from build123d import *

# Parameters (mm, degrees)
F0_R     = 171.45
F0_R_2   = 19.05
F0_R_3   = 6.35
F1_DEPTH = 31.75
F2_DEPTH = 6.35


with BuildPart() as f1:
    # F0 (on Front) → F1 (new body)
    with BuildSketch(Plane.XZ):
        Circle(F0_R)
        with Locations((0, -50.8)):
            Circle(F0_R_2, mode=Mode.SUBTRACT)
        with Locations((-50.8, 0)):
            Circle(F0_R_2, mode=Mode.SUBTRACT)
        Circle(F0_R_3, mode=Mode.SUBTRACT)
        with Locations((50.8, 0)):
            Circle(F0_R_2, mode=Mode.SUBTRACT)
        with Locations((0, 50.8)):
            Circle(F0_R_2, mode=Mode.SUBTRACT)
    extrude(amount=F1_DEPTH)

    # F0 (on Front) → F2 (join)
    with BuildSketch(Plane.XZ):
        with Locations((0, 50.8)):
            Circle(F0_R_2)
        with Locations((50.8, 0)):
            Circle(F0_R_2)
        with Locations((-50.8, 0)):
            Circle(F0_R_2)
        with Locations((0, -50.8)):
            Circle(F0_R_2)
    extrude(amount=F2_DEPTH)


solid = f1.part
Read the model definition and answer for the solid it produces. Units are mm, in the model's axes. A direction names the side the tool comes from. Coordinates: 2 decimals unless noted, no trailing zeros. Loops run counter-clockwise (first coordinate to the right, second up) from the corner with the lowest first, then second, coordinate; pieces in that order, holes last. Notation, with made-up numbers: (-2, 86) -> (5, 86) arc R21 cw to (5, 107) -> close; hole circle Ø4 at (46.5, 80.5). An arc over 180 degrees is marked (long way). Answer in a Markdown table with one row per item.
Item 1: For a pull along X with two mould halves and no side action, classify faces 3 (the cylindrical face through (92.17, -15.653, 144.567)), 4 (the cylindrical face through (-4.13, -18.872, 32.203)), 5 (the flat face through (36, 0, 2)) as released by +X, released by -X, zero draft, split by the parting line, or undercut.
Returned:
| item | result |
|---|---|
| face 3 | split by the parting line |
| face 4 | undercut |
| face 5 | zero draft |
Item 2: For faces 1 (the flat face through (36, -31.75, -36)), 2 (the flat face through (0, -6.35, -51)), determine the directions among +Z, -Z, +X, -X, +Y, -Y from which every point of the face is accessible in a straight line to the end or side of a thin tool.
Returned:
| item | result |
|---|---|
| face 1 | +Z, -Z, +X, -X, -Y |
| face 2 | -Y |
Item 3: A cutting plane is placed at C-C on z = 50.8. Determine the outline of the cut face in (x, y).
Returned:
| item | result |
|---|---|
| outline | (-163.75, -31.75) -> (-19.05, -31.75) -> (-19.05, -6.35) -> (19.05, -6.35) -> (19.05, -31.75) -> (163.75, -31.75) -> (163.75, 0) -> (-163.75, 0) -> close |
Item 4: Each of these flat-tipped pins is pushed along its axis until it touches: P1, Ø19, axis at x = -8, z = -53, coming from the -Y side; P2, Ø10, axis at y = -13.5, z = 23, coming from the -X side; P3, Ø2, axis at x = 87, y = -12, coming from the +Z side. Where does it stop, or does it pass through?
Returned:
| item | result |
|---|---|
| P1 | stops at y = -6.35 |
| P2 | stops at x = -170.5 |
| P3 | stops at z = 148.32 |
Item 5: A cutting plane is placed at B-B on y = -17. Determine the outline of the cut face in (x, z).
Returned:
| item | result |
|---|---|
| outline | circle Ø342.9 at (0, 0); hole circle Ø38.1 at (-50.8, 0); hole circle Ø38.1 at (0, -50.8); hole circle Ø38.1 at (0, 50.8); hole circle Ø12.7 at (0, 0); hole circle Ø38.1 at (50.8, 0) |
Item 6: Straight lines are drawn through the part: line 1 along Z through (x, y) = (0, -25.25); line 2 along X through (y, z) = (-23, -43); line 3 along X through (y, z) = (-18.5, -62.5). For each, find the intervals that lie inside material, in ascending order. Write a range as [from, to].
Returned:
| item | result |
|---|---|
| line 1 | z = [-171.45, -69.85], [-31.75, -6.35], [6.35, 31.75], [69.85, 171.45] |
| line 2 | x = [-165.97, -17.38], [17.38, 165.97] |
| line 3 | x = [-159.65, -15.03], [15.03, 159.65] |
Item 7: A cutting plane is placed at A-A on x = 0. Determine the outline of the cut face in (y, z), plus the area to 3 significant figures.
Returned:
| item | result |
|---|---|
| outline | (-31.75, -171.45) -> (0, -171.45) -> (0, -6.35) -> (-31.75, -6.35) -> (-31.75, -31.75) -> (-6.35, -31.75) -> (-6.35, -69.85) -> (-31.75, -69.85) -> close; (-31.75, 6.35) -> (0, 6.35) -> (0, 171.45) -> (-31.75, 171.45) -> (-31.75, 69.85) -> (-6.35, 69.85) -> (-6.35, 31.75) -> (-31.75, 31.75) -> close |
| area | 8,550 mm^2 |
Item 8: A cutting plane is placed at D-D on x = -44.5. Determine the outline of the cut face in (y, z), plus the area to 3 significant figures.
Returned:
| item | result |
|---|---|
| outline | (-31.75, -165.57) -> (0, -165.57) -> (0, 165.57) -> (-31.75, 165.57) -> (-31.75, 17.98) -> (-6.35, 17.98) -> (-6.35, -17.98) -> (-31.75, -17.98) -> close |
| area | 9,600 mm^2 |
